Part model, mm, in its own coordinate system. Face numbers are marked on the shaded views. A direction names the side the tool comes from. Give positions to 0.01 mm unless a question says otherwise; leave off trailing zeros. Answer as a JSON object with one key per item and string values.
from build123d import *

# Parameters (mm, degrees)
CROQUIS2_W                          = 25.5
CROQUIS2_H                          = 10.1
SALIENTE_EXTRUIR2_DEPTH             = 7.9
CORTAR_EXTRUIR1_DEPTH               = 26.5
CROQUIS4_W                          = 1.74
CROQUIS4_H                          = 5
SALIENTE_EXTRUIR3_DEPTH             = 0.1
CORTAR_EXTRUIR2_DEPTH               = 11.1
CROQUIS7_R                          = 0.225
SALIENTE_EXTRUIR4_DEPTH             = 7
SALIENTE_EXTRUIR4_DIRECTION_2_REACH = 10


with BuildPart() as part:
    # Croquis2 → Saliente-Extruir2 (new body)
    with BuildSketch(Plane(origin=(0, 0, 0), x_dir=(1, 0, 0), z_dir=(0, 1, 0))):
        with Locations((12.75, 5.05)):
            Rectangle(CROQUIS2_W, CROQUIS2_H)
    extrude(amount=SALIENTE_EXTRUIR2_DEPTH)

    # Croquis3 → Cortar-Extruir1 (cut, through all)
    with BuildSketch(Plane(origin=(25.5, 0, 0), x_dir=(0, 0, -1), z_dir=(1, 0, 0))):
        Polygon((1.55, 0), (2.55, 1), (7.55, 1), (8.55, 0), align=None)
    extrude(amount=-CORTAR_EXTRUIR1_DEPTH, mode=Mode.SUBTRACT)

    # Croquis4 → Saliente-Extruir3 (add)
    with BuildSketch(Plane(origin=(0, 7.9, 0), x_dir=(1, 0, 0), z_dir=(0, 1, 0))):
        with Locations((1.32, 5.05)):
            Rectangle(CROQUIS4_W, CROQUIS4_H)
        with Locations((3.86, 5.05)):
            Rectangle(CROQUIS4_W, CROQUIS4_H)
        with Locations((6.4, 5.05)):
            Rectangle(CROQUIS4_W, CROQUIS4_H)
        with Locations((8.94, 5.05)):
            Rectangle(CROQUIS4_W, CROQUIS4_H)
        with Locations((11.48, 5.05)):
            Rectangle(CROQUIS4_W, CROQUIS4_H)
        with Locations((14.02, 5.05)):
            Rectangle(CROQUIS4_W, CROQUIS4_H)
        with Locations((16.56, 5.05)):
            Rectangle(CROQUIS4_W, CROQUIS4_H)
        with Locations((19.1, 5.05)):
            Rectangle(CROQUIS4_W, CROQUIS4_H)
        with Locations((21.64, 5.05)):
            Rectangle(CROQUIS4_W, CROQUIS4_H)
        with Locations((24.18, 5.05)):
            Rectangle(CROQUIS4_W, CROQUIS4_H)
    extrude(amount=SALIENTE_EXTRUIR3_DEPTH)

    # Croquis6 → Cortar-Extruir2 (cut, through all)
    with BuildSketch(Plane(origin=(0, 0, -10.1), x_dir=(-1, 0, 0), z_dir=(0, 0, -1))):
        Polygon((-23.18, 1), (-24.18, 0), (-1.32, 0), (-2.32, 1), align=None)
    extrude(amount=-CORTAR_EXTRUIR2_DEPTH, mode=Mode.SUBTRACT)

    # Croquis7 → Saliente-Extruir4 (add)
    with BuildSketch(Plane.XZ):
        with Locations((1.32, -8.86)):
            Circle(CROQUIS7_R)
        with Locations((3.86, -8.86)):
            Circle(CROQUIS7_R)
        with Locations((6.4, -8.86)):
            Circle(CROQUIS7_R)
        with Locations((8.94, -8.86)):
            Circle(CROQUIS7_R)
        with Locations((11.48, -8.86)):
            Circle(CROQUIS7_R)
        with Locations((14.02, -8.86)):
            Circle(CROQUIS7_R)
        with Locations((16.56, -8.86)):
            Circle(CROQUIS7_R)
        with Locations((19.1, -8.86)):
            Circle(CROQUIS7_R)
        with Locations((21.64, -8.86)):
            Circle(CROQUIS7_R)
        with Locations((24.18, -8.86)):
            Circle(CROQUIS7_R)
        with Locations((3.86, -1.24)):
            Circle(CROQUIS7_R)
        with Locations((6.4, -1.24)):
            Circle(CROQUIS7_R)
        with Locations((8.94, -1.24)):
            Circle(CROQUIS7_R)
        with Locations((11.48, -1.24)):
            Circle(CROQUIS7_R)
        with Locations((14.02, -1.24)):
            Circle(CROQUIS7_R)
        with Locations((16.56, -1.24)):
            Circle(CROQUIS7_R)
        with Locations((19.1, -1.24)):
            Circle(CROQUIS7_R)
        with Locations((21.64, -1.24)):
            Circle(CROQUIS7_R)
        with Locations((24.18, -1.24)):
            Circle(CROQUIS7_R)
        with Locations((1.32, -1.24)):
            Circle(CROQUIS7_R)
    extrude(amount=SALIENTE_EXTRUIR4_DEPTH)

    # Croquis7 → Saliente-Extruir4 direction 2 (add, up to next)
    with BuildSketch(Plane.XZ, mode=Mode.PRIVATE) as saliente_extruir4_direction_2_sk1:
        with Locations((1.32, -8.86)):
            Circle(CROQUIS7_R)
    saliente_extruir4_direction_2_tool1 = extrude(saliente_extruir4_direction_2_sk1.sketch, amount=-SALIENTE_EXTRUIR4_DIRECTION_2_REACH, mode=Mode.PRIVATE) - part.part
    add(saliente_extruir4_direction_2_tool1.solids().sort_by_distance((1.32, 0, -8.86))[0])
    # Croquis7 → Saliente-Extruir4 direction 2 (add, up to next)
    with BuildSketch(Plane.XZ, mode=Mode.PRIVATE) as saliente_extruir4_direction_2_sk2:
        with Locations((3.86, -8.86)):
            Circle(CROQUIS7_R)
    saliente_extruir4_direction_2_tool2 = extrude(saliente_extruir4_direction_2_sk2.sketch, amount=-SALIENTE_EXTRUIR4_DIRECTION_2_REACH, mode=Mode.PRIVATE) - part.part
    add(saliente_extruir4_direction_2_tool2.solids().sort_by_distance((3.86, 0, -8.86))[0])
    # Croquis7 → Saliente-Extruir4 direction 2 (add, up to next)
    with BuildSketch(Plane.XZ, mode=Mode.PRIVATE) as saliente_extruir4_direction_2_sk3:
        with Locations((6.4, -8.86)):
            Circle(CROQUIS7_R)
    saliente_extruir4_direction_2_tool3 = extrude(saliente_extruir4_direction_2_sk3.sketch, amount=-SALIENTE_EXTRUIR4_DIRECTION_2_REACH, mode=Mode.PRIVATE) - part.part
    add(saliente_extruir4_direction_2_tool3.solids().sort_by_distance((6.4, 0, -8.86))[0])
    # Croquis7 → Saliente-Extruir4 direction 2 (add, up to next)
    with BuildSketch(Plane.XZ, mode=Mode.PRIVATE) as saliente_extruir4_direction_2_sk4:
        with Locations((8.94, -8.86)):
            Circle(CROQUIS7_R)
    saliente_extruir4_direction_2_tool4 = extrude(saliente_extruir4_direction_2_sk4.sketch, amount=-SALIENTE_EXTRUIR4_DIRECTION_2_REACH, mode=Mode.PRIVATE) - part.part
    add(saliente_extruir4_direction_2_tool4.solids().sort_by_distance((8.94, 0, -8.86))[0])
    # Croquis7 → Saliente-Extruir4 direction 2 (add, up to next)
    with BuildSketch(Plane.XZ, mode=Mode.PRIVATE) as saliente_extruir4_direction_2_sk5:
        with Locations((11.48, -8.86)):
            Circle(CROQUIS7_R)
    saliente_extruir4_direction_2_tool5 = extrude(saliente_extruir4_direction_2_sk5.sketch, amount=-SALIENTE_EXTRUIR4_DIRECTION_2_REACH, mode=Mode.PRIVATE) - part.part
    add(saliente_extruir4_direction_2_tool5.solids().sort_by_distance((11.48, 0, -8.86))[0])
    # Croquis7 → Saliente-Extruir4 direction 2 (add, up to next)
    with BuildSketch(Plane.XZ, mode=Mode.PRIVATE) as saliente_extruir4_direction_2_sk6:
        with Locations((14.02, -8.86)):
            Circle(CROQUIS7_R)
    saliente_extruir4_direction_2_tool6 = extrude(saliente_extruir4_direction_2_sk6.sketch, amount=-SALIENTE_EXTRUIR4_DIRECTION_2_REACH, mode=Mode.PRIVATE) - part.part
    add(saliente_extruir4_direction_2_tool6.solids().sort_by_distance((14.02, 0, -8.86))[0])
    # Croquis7 → Saliente-Extruir4 direction 2 (add, up to next)
    with BuildSketch(Plane.XZ, mode=Mode.PRIVATE) as saliente_extruir4_direction_2_sk7:
        with Locations((16.56, -8.86)):
            Circle(CROQUIS7_R)
    saliente_extruir4_direction_2_tool7 = extrude(saliente_extruir4_direction_2_sk7.sketch, amount=-SALIENTE_EXTRUIR4_DIRECTION_2_REACH, mode=Mode.PRIVATE) - part.part
    add(saliente_extruir4_direction_2_tool7.solids().sort_by_distance((16.56, 0, -8.86))[0])
    # Croquis7 → Saliente-Extruir4 direction 2 (add, up to next)
    with BuildSketch(Plane.XZ, mode=Mode.PRIVATE) as saliente_extruir4_direction_2_sk8:
        with Locations((19.1, -8.86)):
            Circle(CROQUIS7_R)
    saliente_extruir4_direction_2_tool8 = extrude(saliente_extruir4_direction_2_sk8.sketch, amount=-SALIENTE_EXTRUIR4_DIRECTION_2_REACH, mode=Mode.PRIVATE) - part.part
    add(saliente_extruir4_direction_2_tool8.solids().sort_by_distance((19.1, 0, -8.86))[0])
    # Croquis7 → Saliente-Extruir4 direction 2 (add, up to next)
    with BuildSketch(Plane.XZ, mode=Mode.PRIVATE) as saliente_extruir4_direction_2_sk9:
        with Locations((21.64, -8.86)):
            Circle(CROQUIS7_R)
    saliente_extruir4_direction_2_tool9 = extrude(saliente_extruir4_direction_2_sk9.sketch, amount=-SALIENTE_EXTRUIR4_DIRECTION_2_REACH, mode=Mode.PRIVATE) - part.part
    add(saliente_extruir4_direction_2_tool9.solids().sort_by_distance((21.64, 0, -8.86))[0])
    # Croquis7 → Saliente-Extruir4 direction 2 (add, up to next)
    with BuildSketch(Plane.XZ, mode=Mode.PRIVATE) as saliente_extruir4_direction_2_sk10:
        with Locations((24.18, -8.86)):
            Circle(CROQUIS7_R)
    saliente_extruir4_direction_2_tool10 = extrude(saliente_extruir4_direction_2_sk10.sketch, amount=-SALIENTE_EXTRUIR4_DIRECTION_2_REACH, mode=Mode.PRIVATE) - part.part
    add(saliente_extruir4_direction_2_tool10.solids().sort_by_distance((24.18, 0, -8.86))[0])
    # Croquis7 → Saliente-Extruir4 direction 2 (add, up to next)
    with BuildSketch(Plane.XZ, mode=Mode.PRIVATE) as saliente_extruir4_direction_2_sk11:
        with Locations((3.86, -1.24)):
            Circle(CROQUIS7_R)
    saliente_extruir4_direction_2_tool11 = extrude(saliente_extruir4_direction_2_sk11.sketch, amount=-SALIENTE_EXTRUIR4_DIRECTION_2_REACH, mode=Mode.PRIVATE) - part.part
    add(saliente_extruir4_direction_2_tool11.solids().sort_by_distance((3.86, 0, -1.24))[0])
    # Croquis7 → Saliente-Extruir4 direction 2 (add, up to next)
    with BuildSketch(Plane.XZ, mode=Mode.PRIVATE) as saliente_extruir4_direction_2_sk12:
        with Locations((6.4, -1.24)):
            Circle(CROQUIS7_R)
    saliente_extruir4_direction_2_tool12 = extrude(saliente_extruir4_direction_2_sk12.sketch, amount=-SALIENTE_EXTRUIR4_DIRECTION_2_REACH, mode=Mode.PRIVATE) - part.part
    add(saliente_extruir4_direction_2_tool12.solids().sort_by_distance((6.4, 0, -1.24))[0])
    # Croquis7 → Saliente-Extruir4 direction 2 (add, up to next)
    with BuildSketch(Plane.XZ, mode=Mode.PRIVATE) as saliente_extruir4_direction_2_sk13:
        with Locations((8.94, -1.24)):
            Circle(CROQUIS7_R)
    saliente_extruir4_direction_2_tool13 = extrude(saliente_extruir4_direction_2_sk13.sketch, amount=-SALIENTE_EXTRUIR4_DIRECTION_2_REACH, mode=Mode.PRIVATE) - part.part
    add(saliente_extruir4_direction_2_tool13.solids().sort_by_distance((8.94, 0, -1.24))[0])
    # Croquis7 → Saliente-Extruir4 direction 2 (add, up to next)
    with BuildSketch(Plane.XZ, mode=Mode.PRIVATE) as saliente_extruir4_direction_2_sk14:
        with Locations((11.48, -1.24)):
            Circle(CROQUIS7_R)
    saliente_extruir4_direction_2_tool14 = extrude(saliente_extruir4_direction_2_sk14.sketch, amount=-SALIENTE_EXTRUIR4_DIRECTION_2_REACH, mode=Mode.PRIVATE) - part.part
    add(saliente_extruir4_direction_2_tool14.solids().sort_by_distance((11.48, 0, -1.24))[0])
    # Croquis7 → Saliente-Extruir4 direction 2 (add, up to next)
    with BuildSketch(Plane.XZ, mode=Mode.PRIVATE) as saliente_extruir4_direction_2_sk15:
        with Locations((14.02, -1.24)):
            Circle(CROQUIS7_R)
    saliente_extruir4_direction_2_tool15 = extrude(saliente_extruir4_direction_2_sk15.sketch, amount=-SALIENTE_EXTRUIR4_DIRECTION_2_REACH, mode=Mode.PRIVATE) - part.part
    add(saliente_extruir4_direction_2_tool15.solids().sort_by_distance((14.02, 0, -1.24))[0])
    # Croquis7 → Saliente-Extruir4 direction 2 (add, up to next)
    with BuildSketch(Plane.XZ, mode=Mode.PRIVATE) as saliente_extruir4_direction_2_sk16:
        with Locations((16.56, -1.24)):
            Circle(CROQUIS7_R)
    saliente_extruir4_direction_2_tool16 = extrude(saliente_extruir4_direction_2_sk16.sketch, amount=-SALIENTE_EXTRUIR4_DIRECTION_2_REACH, mode=Mode.PRIVATE) - part.part
    add(saliente_extruir4_direction_2_tool16.solids().sort_by_distance((16.56, 0, -1.24))[0])
    # Croquis7 → Saliente-Extruir4 direction 2 (add, up to next)
    with BuildSketch(Plane.XZ, mode=Mode.PRIVATE) as saliente_extruir4_direction_2_sk17:
        with Locations((19.1, -1.24)):
            Circle(CROQUIS7_R)
    saliente_extruir4_direction_2_tool17 = extrude(saliente_extruir4_direction_2_sk17.sketch, amount=-SALIENTE_EXTRUIR4_DIRECTION_2_REACH, mode=Mode.PRIVATE) - part.part
    add(saliente_extruir4_direction_2_tool17.solids().sort_by_distance((19.1, 0, -1.24))[0])
    # Croquis7 → Saliente-Extruir4 direction 2 (add, up to next)
    with BuildSketch(Plane.XZ, mode=Mode.PRIVATE) as saliente_extruir4_direction_2_sk18:
        with Locations((21.64, -1.24)):
            Circle(CROQUIS7_R)
    saliente_extruir4_direction_2_tool18 = extrude(saliente_extruir4_direction_2_sk18.sketch, amount=-SALIENTE_EXTRUIR4_DIRECTION_2_REACH, mode=Mode.PRIVATE) - part.part
    add(saliente_extruir4_direction_2_tool18.solids().sort_by_distance((21.64, 0, -1.24))[0])
    # Croquis7 → Saliente-Extruir4 direction 2 (add, up to next)
    with BuildSketch(Plane.XZ, mode=Mode.PRIVATE) as saliente_extruir4_direction_2_sk19:
        with Locations((24.18, -1.24)):
            Circle(CROQUIS7_R)
    saliente_extruir4_direction_2_tool19 = extrude(saliente_extruir4_direction_2_sk19.sketch, amount=-SALIENTE_EXTRUIR4_DIRECTION_2_REACH, mode=Mode.PRIVATE) - part.part
    add(saliente_extruir4_direction_2_tool19.solids().sort_by_distance((24.18, 0, -1.24))[0])
    # Croquis7 → Saliente-Extruir4 direction 2 (add, up to next)
    with BuildSketch(Plane.XZ, mode=Mode.PRIVATE) as saliente_extruir4_direction_2_sk20:
        with Locations((1.32, -1.24)):
            Circle(CROQUIS7_R)
    saliente_extruir4_direction_2_tool20 = extrude(saliente_extruir4_direction_2_sk20.sketch, amount=-SALIENTE_EXTRUIR4_DIRECTION_2_REACH, mode=Mode.PRIVATE) - part.part
    add(saliente_extruir4_direction_2_tool20.solids().sort_by_distance((1.32, 0, -1.24))[0])


solid = part.part
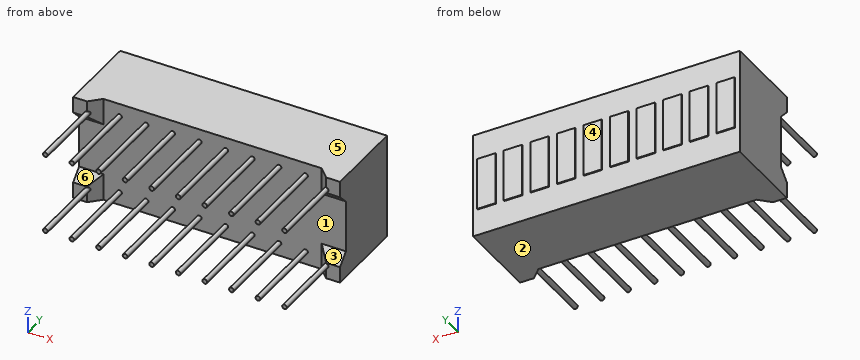
1. Pin check, flat tips, straight feed: P1, Ø3, axis at y = -3.5, z = -2.5, coming from the -X side (3 decimals); P2, Ø0.7, axis at x = 0.5, z = -0.5, coming from the -Y side. Stop position of each tip, or through.
Worked answers:
{"P1": "stops at x = 1.095", "P2": "stops at y = 0"}
2. Which spindle directions (+Z, -Z, +X, -X, +Y, -Y) get a long thin tool onto all of the face, cutting with end or side? Do the marked faces 1, 2 and 3. Say none if no direction does.
Worked answers:
{"face 1": "-Y", "face 2": "-Z, +X, -X, +Y, -Y", "face 3": "+X, -X, -Y"}
3. Two-plate mould, pull along Z, no slides. Class the marked faces 4, 5 and 6: +Z half, -Z half, draft (parallel to the pull), parting line (faces both ways), or undercut.
Worked answers:
{"face 4": "draft", "face 5": "+Z half", "face 6": "undercut"}
4. Probe line 1 along Y through (x, z) = (21.5, -6.75); line 2 along Y through (x, z) = (10, -2); line 3 along Z through (x, y) = (6.5, -0.75). List the from-to ranges inside material, lowest first.
Worked answers:
{"line 1": "y = 1 to 8", "line 2": "y = 1 to 7.9", "line 3": "z = -9.06 to -8.66, -1.44 to -1.04"}
